```python
from build123d import *

# Parameters (mm, degrees)
SKETCH1_W           = 98
SKETCH1_H           = 65
BOSS_EXTRUDE1_DEPTH = 32
SKETCH2_R           = 14.5
CUT_EXTRUDE1_DEPTH  = 27
FILLET1_R           = 10
FILLET2_R           = 10
FILLET3_R           = 10
FILLET4_R           = 10
CHAMFER1_SIZE       = 2
CUT_EXTRUDE2_START  = -0.5
SKETCH3_W           = 60
SKETCH3_H           = 10
CUT_EXTRUDE2_DEPTH  = 3


with BuildPart() as part:
    # Sketch1 → Boss-Extrude1 (new body)
    with BuildSketch(Plane(origin=(0, 0, 0), x_dir=(1, 0, 0), z_dir=(0, 1, 0))):
        with Locations((-41, -4.919354839)):
            Rectangle(SKETCH1_W, SKETCH1_H)
    extrude(amount=BOSS_EXTRUDE1_DEPTH)

    # Sketch2 → Cut-Extrude1 (cut)
    with BuildSketch(Plane(origin=(0, 32, 0), x_dir=(1, 0, 0), z_dir=(0, 1, 0))):
        with Locations(Location((-16.5, 11.330645161, 0), (0, 0, 270))):
            Circle(SKETCH2_R)
        with Locations(Location((-16.5, -21.169354839, 0), (0, 0, 90))):
            Circle(SKETCH2_R)
        with Locations(Location((-65.5, 11.330645161, 0), (0, 0, 90))):
            Circle(SKETCH2_R)
        with Locations(Location((-65.5, -21.169354839, 0), (0, 0, 270))):
            Circle(SKETCH2_R)
    extrude(amount=-CUT_EXTRUDE1_DEPTH, mode=Mode.SUBTRACT)

    # Fillet1
    fillet1_edges = [part.edges().sort_by_distance(p)[0] for p in [
        (8, 16, -27.580645161),
    ]]
    fillet(fillet1_edges, radius=FILLET1_R)

    # Fillet2
    fillet2_edges = [part.edges().sort_by_distance(p)[0] for p in [
        (-90, 16, 37.419354839),
    ]]
    fillet(fillet2_edges, radius=FILLET2_R)

    # Fillet3
    fillet3_edges = [part.edges().sort_by_distance(p)[0] for p in [
        (-90, 16, -27.580645161),
    ]]
    fillet(fillet3_edges, radius=FILLET3_R)

    # Fillet4
    fillet4_edges = [part.edges().sort_by_distance(p)[0] for p in [
        (8, 16, 37.419354839),
    ]]
    fillet(fillet4_edges, radius=FILLET4_R)

    # Chamfer1
    # the kernel refuses this chamfer: 2 mm, written as the material it adds along each edge
    with BuildSketch(Plane(origin=(-16.5, 5, 21.169354839), x_dir=(0, 0, -1), z_dir=(1, 0, 0))) as chamfer1_piece_1:
        Polygon((14.5, CHAMFER1_SIZE), (14.5 - CHAMFER1_SIZE, 0), (14.5, 0), align=None)
    revolve(axis=Axis((-16.5, 5, 21.169354839), (0, 1, 0)))
    with BuildSketch(Plane(origin=(-65.5, 5, -11.330645161), x_dir=(0, 0, -1), z_dir=(1, 0, 0))) as chamfer1_piece_2:
        Polygon((14.5, CHAMFER1_SIZE), (14.5 - CHAMFER1_SIZE, 0), (14.5, 0), align=None)
    revolve(axis=Axis((-65.5, 5, -11.330645161), (0, 1, 0)))
    with BuildSketch(Plane(origin=(-65.5, 5, 21.169354839), x_dir=(0, 0, 1), z_dir=(-1, 0, 0))) as chamfer1_piece_3:
        Polygon((14.5, CHAMFER1_SIZE), (14.5 - CHAMFER1_SIZE, 0), (14.5, 0), align=None)
    revolve(axis=Axis((-65.5, 5, 21.169354839), (0, 1, 0)))
    with BuildSketch(Plane(origin=(-16.5, 5, -11.330645161), x_dir=(0, 0, 1), z_dir=(-1, 0, 0))) as chamfer1_piece_4:
        Polygon((14.5, CHAMFER1_SIZE), (14.5 - CHAMFER1_SIZE, 0), (14.5, 0), align=None)
    revolve(axis=Axis((-16.5, 5, -11.330645161), (0, 1, 0)))
    # the kernel refuses this chamfer: 2 mm, written as the material it takes off along each edge
    with BuildSketch(Plane(origin=(-16.5, 32, 21.169354839), x_dir=(0, 0, -1), z_dir=(1, 0, 0))) as chamfer1_2_piece_1:
        Polygon((14.5 + CHAMFER1_SIZE, 0), (14.5, -CHAMFER1_SIZE), (14.5, 0), align=None)
    revolve(axis=Axis((-16.5, 32, 21.169354839), (0, 1, 0)), mode=Mode.SUBTRACT)
    with BuildSketch(Plane(origin=(-65.5, 32, -11.330645161), x_dir=(0, 0, -1), z_dir=(1, 0, 0))) as chamfer1_2_piece_2:
        Polygon((14.5 + CHAMFER1_SIZE, 0), (14.5, -CHAMFER1_SIZE), (14.5, 0), align=None)
    revolve(axis=Axis((-65.5, 32, -11.330645161), (0, 1, 0)), mode=Mode.SUBTRACT)
    with BuildSketch(Plane(origin=(-65.5, 32, 21.169354839), x_dir=(0, 0, 1), z_dir=(-1, 0, 0))) as chamfer1_2_piece_3:
        Polygon((14.5 + CHAMFER1_SIZE, 0), (14.5, -CHAMFER1_SIZE), (14.5, 0), align=None)
    revolve(axis=Axis((-65.5, 32, 21.169354839), (0, 1, 0)), mode=Mode.SUBTRACT)
    with BuildSketch(Plane(origin=(-16.5, 32, -11.330645161), x_dir=(0, 0, 1), z_dir=(-1, 0, 0))) as chamfer1_2_piece_4:
        Polygon((14.5 + CHAMFER1_SIZE, 0), (14.5, -CHAMFER1_SIZE), (14.5, 0), align=None)
    revolve(axis=Axis((-16.5, 32, -11.330645161), (0, 1, 0)), mode=Mode.SUBTRACT)
    with BuildSketch(Plane(origin=(-80, 0, -27.580645161), x_dir=(0, -0.02749587661058639, 0.9996219169112968), z_dir=(1, 0, 0)), Plane(origin=(-80, 32, -27.580645161), x_dir=(0, -0.9996219169112968, -0.027495876610585647), z_dir=(1, 0, 0)), Plane(origin=(-2, 0, 37.419354839), x_dir=(0, -0.02749587661058639, -0.9996219169112968), z_dir=(-1, 0, 0)), Plane(origin=(-2, 32, 37.419354839), x_dir=(0, -0.9996219169112968, 0.027495876610585647), z_dir=(-1, 0, 0))) as chamfer1_2_piece_5:
        Polygon((CHAMFER1_SIZE * 0.999621916911, -CHAMFER1_SIZE * 0.0274958766106), (-CHAMFER1_SIZE * 0.0274958766106, -CHAMFER1_SIZE * 0.999621916911), (0, 0), align=None)
    extrude(amount=78, mode=Mode.SUBTRACT)
    with BuildSketch(Plane(origin=(-2, 0, -17.580645161), x_dir=(0, 0, -1), z_dir=(-1, 0, 0))) as chamfer1_2_piece_6:
        Polygon((10 - CHAMFER1_SIZE, 0), (10, -CHAMFER1_SIZE), (10, 0), align=None)
    revolve(axis=Axis((-2, 0, -17.580645161), (0, -1, 0)), revolution_arc=90, mode=Mode.SUBTRACT)
    with BuildSketch(Plane(origin=(-2, 32, -17.580645161), x_dir=(0, 0, -1), z_dir=(-1, 0, 0))) as chamfer1_2_piece_7:
        Polygon((10, CHAMFER1_SIZE), (10 - CHAMFER1_SIZE, 0), (10, 0), align=None)
    revolve(axis=Axis((-2, 32, -17.580645161), (0, -1, 0)), revolution_arc=90, mode=Mode.SUBTRACT)
    with BuildSketch(Plane(origin=(-80, 32, 27.419354839), x_dir=(-1, 0, 0), z_dir=(0, 0, -1))) as chamfer1_2_piece_8:
        Polygon((10, -CHAMFER1_SIZE), (10 - CHAMFER1_SIZE, 0), (10, 0), align=None)
    revolve(axis=Axis((-80, 32, 27.419354839), (0, 1, 0)), revolution_arc=90, mode=Mode.SUBTRACT)
    with BuildSketch(Plane(origin=(-80, 0, 27.419354839), x_dir=(-1, 0, 0), z_dir=(0, 0, -1))) as chamfer1_2_piece_9:
        Polygon((10 - CHAMFER1_SIZE, 0), (10, CHAMFER1_SIZE), (10, 0), align=None)
    revolve(axis=Axis((-80, 0, 27.419354839), (0, 1, 0)), revolution_arc=90, mode=Mode.SUBTRACT)
    with BuildSketch(Plane(origin=(-90, 0, 27.419354839), x_dir=(0.9996219169112968, -0.027495876610586292, 0), z_dir=(0, 0, -1)), Plane(origin=(-90, 32, 27.419354839), x_dir=(-0.0274958766105891, -0.9996219169112968, 0), z_dir=(0, 0, -1)), Plane(origin=(8, 0, -17.580645161), x_dir=(-0.9996219169112968, -0.027495876610586438, 0), z_dir=(0, 0, 1)), Plane(origin=(8, 32, -17.580645161), x_dir=(0.02749587661058651, -0.9996219169112968, 0), z_dir=(0, 0, 1))) as chamfer1_2_piece_10:
        Polygon((CHAMFER1_SIZE * 0.999621916911, -CHAMFER1_SIZE * 0.0274958766106), (-CHAMFER1_SIZE * 0.0274958766106, -CHAMFER1_SIZE * 0.999621916911), (0, 0), align=None)
    extrude(amount=45, mode=Mode.SUBTRACT)
    with BuildSketch(Plane(origin=(-80, 0, -17.580645161), x_dir=(-1, 0, 0), z_dir=(0, 0, 1))) as chamfer1_2_piece_11:
        Polygon((10 - CHAMFER1_SIZE, 0), (10, -CHAMFER1_SIZE), (10, 0), align=None)
    revolve(axis=Axis((-80, 0, -17.580645161), (0, -1, 0)), revolution_arc=90, mode=Mode.SUBTRACT)
    with BuildSketch(Plane(origin=(-80, 32, -17.580645161), x_dir=(-1, 0, 0), z_dir=(0, 0, 1))) as chamfer1_2_piece_12:
        Polygon((10, CHAMFER1_SIZE), (10 - CHAMFER1_SIZE, 0), (10, 0), align=None)
    revolve(axis=Axis((-80, 32, -17.580645161), (0, -1, 0)), revolution_arc=90, mode=Mode.SUBTRACT)
    with BuildSketch(Plane(origin=(-2, 32, 27.419354839), x_dir=(0, 0, 1), z_dir=(-1, 0, 0))) as chamfer1_2_piece_13:
        Polygon((10, -CHAMFER1_SIZE), (10 - CHAMFER1_SIZE, 0), (10, 0), align=None)
    revolve(axis=Axis((-2, 32, 27.419354839), (0, 1, 0)), revolution_arc=90, mode=Mode.SUBTRACT)
    with BuildSketch(Plane(origin=(-2, 0, 27.419354839), x_dir=(0, 0, 1), z_dir=(-1, 0, 0))) as chamfer1_2_piece_14:
        Polygon((10 - CHAMFER1_SIZE, 0), (10, CHAMFER1_SIZE), (10, 0), align=None)
    revolve(axis=Axis((-2, 0, 27.419354839), (0, 1, 0)), revolution_arc=90, mode=Mode.SUBTRACT)

    # Sketch3 → Cut-Extrude2 (cut)
    with BuildSketch(Plane.XZ.offset(CUT_EXTRUDE2_START)):
        with Locations((-41, 4.919354839)):
            Rectangle(SKETCH3_W, SKETCH3_H)
    extrude(amount=-CUT_EXTRUDE2_DEPTH, mode=Mode.SUBTRACT)


solid = part.part
```
Geometry: final body of the model. Coordinates: model frame, mm. A direction names the side the tool comes from. Round coordinates to 2 decimals unless told otherwise and drop trailing zeros. Order: outer loops, then holes, each group sorted by start corner. A loop starts at its lowest first (then second) coordinate and runs counter-clockwise, first axis right, second up. Notation, with made-up numbers: (25, 64) -> (35, 64) arc R22 ccw to (35, 85) -> close; hole circle Ø4 at (-24.5, 86.5). An arc over 180 degrees is marked (long way). Use CSV: the item, a comma, the result in double quotes. Start each with the question number.
1) First-contact query: pin 1 Ø23 at (x, z) = (-65.5, 21.17) entering from +Y; pin 2 Ø12.5 at (x, z) = (-69, -5.5) entering from +Y; pin 3 Ø20 at (x, z) = (-68, 27) entering from +Y. Flat tips, straight axial feed; report the tip coordinate or a pass-through.
2) Section A-A (y = 26.5). Return the cut outline in (x, z).
3) Draft query along Z for faces 1 (the face through (-42, 16, -27.581)), 2 (the face through (4.99, 16.2, 34.57)), 3 (the face through (-16, 5, -12)). Return one class per face: +Z half, -Z half, draft (parallel to the pull), parting line (faces both ways), or undercut.
4) Section C-C (x = -16.5). Return the cut outline in (y, z) (3 decimals).
5) Material intervals for line 1 along Z through (x, y) = (-16, 16); line 2 along X through (y, z) = (12, -21.5); line 3 along X through (y, z) = (15, 13.5), sorted ascending. Write a range as from..to.
6) Set-up query: faces 4 (the face through (-2.123, 18.661, -13.218)), 5 (the face through (-41, 0.5, 5)), 6 (the face through (3.99, 0.57, -23.71)). Return all of +Z, -Z, +X, -X, +Y, -Y with unobstructed straight access to the full face (end or side cutting, diameter ignored); none if empty.
7) Section B-B (x = -41.5). Return the cut outline in (y, z).
Returned:
1,pin 1,"stops at y = 5"
1,pin 2,"stops at y = 5.55"
1,pin 3,"stops at y = 31.81"
2,outline,"(-90, -17.58) arc R10 ccw to (-80, -27.58) -> (-2, -27.58) arc R10 ccw to (8, -17.58) -> (8, 27.42) arc R10 ccw to (-2, 37.42) -> (-80, 37.42) arc R10 ccw to (-90, 27.42) -> close; hole circle Ø29 at (-65.5, -11.33); hole circle Ø29 at (-65.5, 21.17); hole circle Ø29 at (-16.5, -11.33); hole circle Ø29 at (-16.5, 21.17)"
3,face 1,"-Z half"
3,face 2,"+Z half"
3,face 3,"undercut"
4,outline,"(0, -25.581) -> (2, -27.581) -> (30, -27.581) -> (30.875, -26.706) -> (30, -25.831) -> (7, -25.831) -> (5, -23.831) -> (5, 1.169) -> (7, 3.169) -> (30, 3.169) -> (31.75, 4.919) -> (30, 6.669) -> (7, 6.669) -> (5, 8.669) -> (5, 33.669) -> (7, 35.669) -> (30, 35.669) -> (30.875, 36.544) -> (30, 37.419) -> (2, 37.419) -> (0, 35.419) -> close; hole (0.5, -0.081) -> (3.5, -0.081) -> (3.5, 9.919) -> (0.5, 9.919) -> close"
5,line 1,"z = -27.58..-25.82, 3.16..6.68, 35.66..37.42"
5,line 2,"x = -89.2..-75.84, -55.16..-26.84, -6.16..7.2"
5,line 3,"x = -90..-77.81, -53.19..-28.81, -4.19..8"
6,face 4,"+Y"
6,face 5,"none"
6,face 6,"-Z, +X, -Y"
7,outline,"(0, -25.58) -> (2, -27.58) -> (30, -27.58) -> (32, -25.58) -> (32, 35.42) -> (30, 37.42) -> (2, 37.42) -> (0, 35.42) -> close; hole (0.5, -0.08) -> (3.5, -0.08) -> (3.5, 9.92) -> (0.5, 9.92) -> close"
